from build123d import *

# Parameters (mm, degrees)
SKETCH_1_W          = 30
SKETCH_1_H          = 38
EXTRUDE_1_DEPTH     = 3
SKETCH_2_R          = 2
CUT_EXTRUDE_1_DEPTH = 3
SKETCH_3_R          = 1.525
CUT_EXTRUDE_2_DEPTH = 3
FILLET_1_R          = 2
SKETCH_4_W          = 20
SKETCH_4_H          = 17
CUT_EXTRUDE_3_DEPTH = 3
FILLET_2_R          = 2


with BuildPart() as part:
    # 草图1 → 凸台-拉伸1 (new body)
    with BuildSketch(Plane.XY):
        Polygon((-45.4, 9.7), (-45.4, -9.7), (-15, -19), (-15, 19), align=None)
        Rectangle(SKETCH_1_W, SKETCH_1_H)
    extrude(amount=EXTRUDE_1_DEPTH)

    # 草图2 → 切除-拉伸1 (cut)
    with BuildSketch(Plane.XY.offset(3)):
        with Locations((0, 12.5)):
            Circle(SKETCH_2_R)
        with Locations((0, -12.5)):
            Circle(SKETCH_2_R)
    extrude(amount=-CUT_EXTRUDE_1_DEPTH, mode=Mode.SUBTRACT)

    # 草图3 → 切除-拉伸2 (cut)
    with BuildSketch(Plane.XY.offset(3)):
        with Locations((-42.9, 5)):
            Circle(SKETCH_3_R)
        with Locations((-27.9, 5)):
            Circle(SKETCH_3_R)
        with Locations((-42.9, -5)):
            Circle(SKETCH_3_R)
        with Locations((-27.9, -5)):
            Circle(SKETCH_3_R)
    extrude(amount=-CUT_EXTRUDE_2_DEPTH, mode=Mode.SUBTRACT)

    # 圆角1
    fillet_1_edges = [part.edges().sort_by_distance(p)[0] for p in [
        (-45.4, 9.7, 1.5),
        (-15, 19, 1.5),
        (15, 19, 1.5),
        (15, -19, 1.5),
        (-15, -19, 1.5),
        (-45.4, -9.7, 1.5),
    ]]
    fillet(fillet_1_edges, radius=FILLET_1_R)

    # 草图4 → 切除-拉伸3 (cut)
    with BuildSketch(Plane.XY.offset(3)):
        Rectangle(SKETCH_4_W, SKETCH_4_H)
    extrude(amount=-CUT_EXTRUDE_3_DEPTH, mode=Mode.SUBTRACT)

    # 圆角2
    fillet_2_edges = [part.edges().sort_by_distance(p)[0] for p in [
        (10, 8.5, 1.5),
        (10, -8.5, 1.5),
        (-10, -8.5, 1.5),
        (-10, 8.5, 1.5),
    ]]
    fillet(fillet_2_edges, radius=FILLET_2_R)


solid = part.part
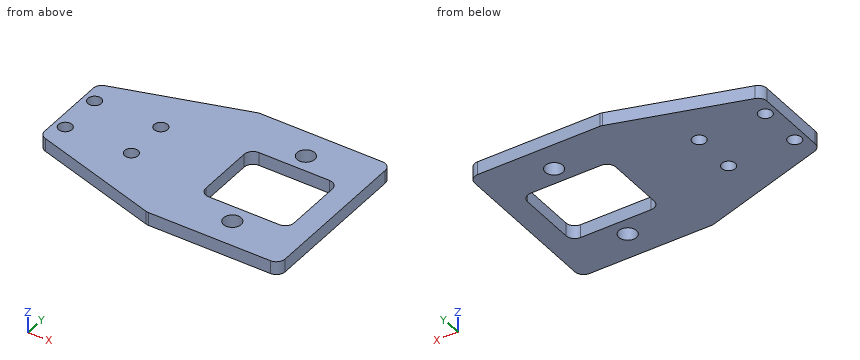
Check sheet for the modelled part. Datum: model origin and axes. Units: mm. Round coordinates to 2 decimals unless told otherwise and drop trailing zeros. Loops run counter-clockwise (first coordinate to the right, second up) from the corner with the lowest first, then second, coordinate; pieces in that order, holes last. Notation, with made-up numbers: (60, -40) - (72, -40) arc R16 cw to (72, -9) - close; hole circle Ø8 at (18, 0.25). An arc over 180 degrees is marked (long way). Answer as CSV lines item,"result". Start each with the question number.
Item 1: Section check C-C (z = 2.2). Count the separate pieces of the cut face and the enclosed holes in it, and give its area (3 significant figures).
Item 2: Section check D-D (y = 5). Record the boundary of the cut face in (x, z) (3 decimals), and give its area (3 significant figures).
Item 3: Section check A-A (x = 0). Record the boundary of the cut face in (y, z), and give its area (3 significant figures).
Item 4: Scan lines: line 1 (Y direction, x = -42.9, z = 1.4) (3 decimals); line 2 (X direction, y = -6, z = 2.8); line 3 (Y direction, x = 4.5, z = 2.5). Record each from-to range of solid material in increasing order. Write a range as [from, to].
Item 5: Section check B-B (y = -2). Record the boundary of the cut face in (x, z), and give its area (3 significant figures).
Report:
1,separate pieces,"1"
1,enclosed holes,"7"
1,area,"1,620 mm2"
2,outline,"(-45.4, 0) - (-44.425, 0) - (-44.425, 3) - (-45.4, 3) - close; (-41.375, 0) - (-29.425, 0) - (-29.425, 3) - (-41.375, 3) - close; (-26.375, 0) - (-10, 0) - (-10, 3) - (-26.375, 3) - close; (10, 0) - (15, 0) - (15, 3) - (10, 3) - close"
2,area,"103 mm2"
3,outline,"(-19, 0) - (-14.5, 0) - (-14.5, 3) - (-19, 3) - close; (-10.5, 0) - (-8.5, 0) - (-8.5, 3) - (-10.5, 3) - close; (8.5, 0) - (10.5, 0) - (10.5, 3) - (8.5, 3) - close; (14.5, 0) - (19, 0) - (19, 3) - (14.5, 3) - close"
3,area,"39.0 mm2"
4,line 1,"y = [-10.465, -6.525], [-3.475, 3.475], [6.525, 10.465]"
4,line 2,"x = [-45.4, -44.05], [-41.75, -29.05], [-26.75, -10], [10, 15]"
4,line 3,"y = [-19, -8.5], [8.5, 19]"
5,outline,"(-45.4, 0) - (-10, 0) - (-10, 3) - (-45.4, 3) - close; (10, 0) - (15, 0) - (15, 3) - (10, 3) - close"
5,area,"121 mm2"
